Could you check a few things on this drawing? It's one solid part, dimensions in mm from its lowest x, y, z. Round coordinates to 2 decimals unless told otherwise and drop trailing zeros. Write each loop counter-clockwise with the first axis right and the second up, starting at its lowest first coordinate (ties: lowest second). Pieces come first, ordered by that corner, then holes. Notation, with made-up numbers: (77.5, 38) -> (132.5, 38) arc R21 cw to (132.5, 63) -> close; hole circle Ø3 at (50, 28). An arc over 180 degrees is marked (long way). Answer in a Markdown table with one row per item.
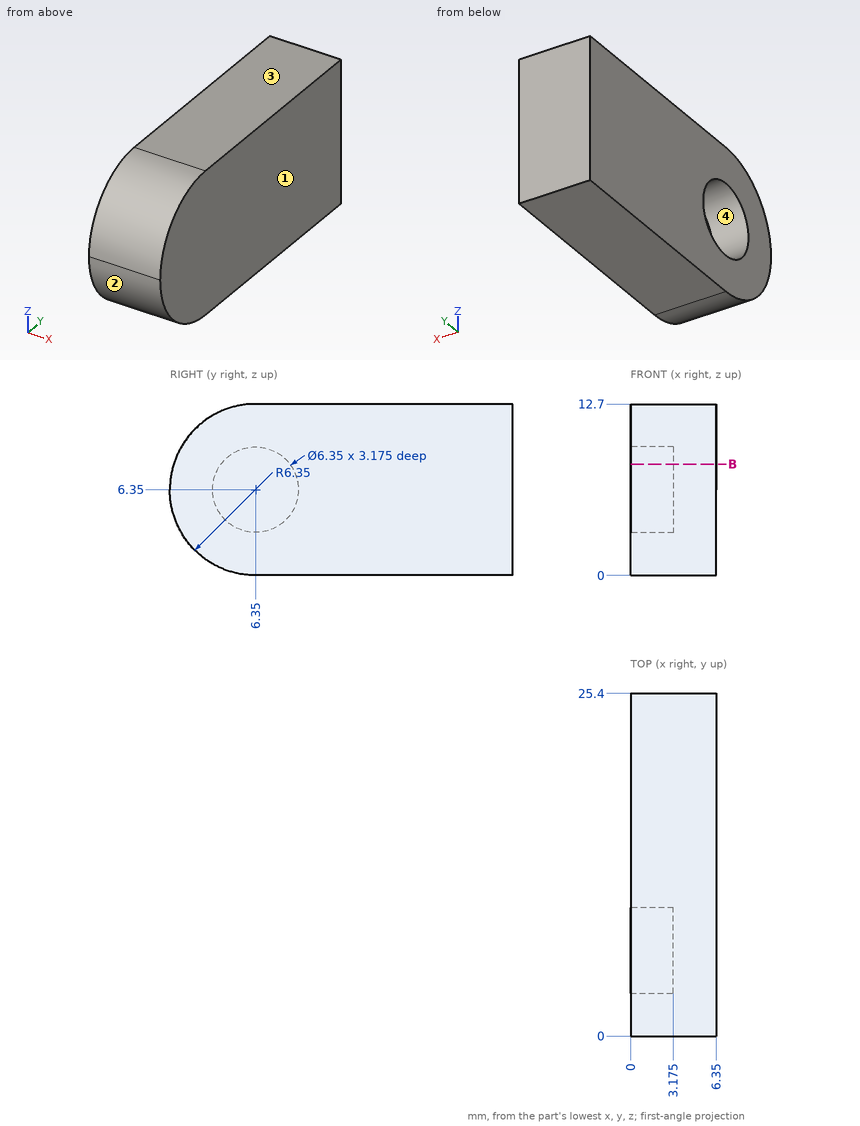
1) Thinking about a two-plate mould opening in Z: for the marked faces 1, 2, 3 and 4, which applies, +Z half, -Z half, draft (parallel to the pull), parting line (faces both ways), or undercut?
Findings:
| item | result |
|---|---|
| face 1 | draft |
| face 2 | -Z half |
| face 3 | +Z half |
| face 4 | undercut |
2) For pin 1 (2 mm diameter, centred on x = 2, y = 3, fed in from -Z); pin 2 (2 mm diameter, centred on x = 4.5, z = 9.5, fed in from -Y) (3 decimals); pin 3 (1.9 mm diameter, centred on y = 7.5, z = 6, fed in from -X) (3 decimals), each with a flat end and sliding along its axis, tell me the tip position at first contact or that it passes through.
Findings:
| item | result |
|---|---|
| pin 1 | stops at z = 0.45 |
| pin 2 | stops at y = 0.375 |
| pin 3 | stops at x = 3.175 |
3) Please list where these lines run through material, in increasing order: line 1 (Z direction, x = 2.1, y = 6.35) (3 decimals); line 2 (X direction, y = 5.5, z = 8.25) (3 decimals); line 3 (Y direction, x = 3.75, z = 1).
Findings:
| item | result |
|---|---|
| line 1 | z = 0 to 3.175, 9.525 to 12.7 |
| line 2 | x = 3.175 to 6.35 |
| line 3 | y = 2.93 to 25.4 |
4) Imagine slicing it at B-B, the plane z = 8.25. Please give me the cut outline in (x, y) (3 decimals), plus the area to 3 significant figures.
Findings:
| item | result |
|---|---|
| outline | (0, 0.291) -> (6.35, 0.291) -> (6.35, 25.4) -> (0, 25.4) -> (0, 8.894) -> (3.175, 8.894) -> (3.175, 3.806) -> (0, 3.806) -> close |
| area | 143 mm^2 |
